Geometry: final body of the model. Coordinates: model frame, mm. Face numbers are marked on the shaded views. A direction names the side the tool comes from. Coordinates: 2 decimals unless noted, no trailing zeros. Order: outer loops, then holes, each group sorted by start corner. A loop starts at its lowest first (then second) coordinate and runs counter-clockwise, first axis right, second up. Notation, with made-up numbers: (-6, 59.5) -> (34, 59.5) arc R16 cw to (34, 85.5) -> close; hole circle Ø2 at (14, 36.25). An arc over 180 degrees is marked (long way). Answer in a Markdown table with one row per item. Add a question column.
1) Contact query for flat-ended pins moving along their axis: P1, Ø1.5, axis at x = 1.5, y = 41.5, coming from the -Z side; P2, Ø15, axis at y = 50, z = 21.5, coming from the -X side; P3, Ø9, axis at y = 52, z = 28, coming from the +X side; P4, Ø4.5, axis at x = 39.94, z = -5.63, coming from the -Y side. Output: stop coordinate, or through.
2) Pull-direction query (Z, two-part tool) for the marked faces 1, 2 and 3; classes: +Z half, -Z half, draft (parallel to the pull), parting line (faces both ways), or undercut.
3) Section query C-C on x = 22.5. Return the cut outline in (y, z).
4) Set-up query: the marked faces 4, 5 and 6. Return all of +Z, -Z, +X, -X, +Y, -Y with unobstructed straight access to the full face (end or side cutting, diameter ignored); none if empty.
5) Ray query, line 1 (X direction, y = 16, z = 21.5); line 2 (X direction, y = 8, z = -7); line 3 (Z direction, x = -11, y = 34.5). Return the intervals inside material, ascending. Write a range as from..to.
6) Section query A-A on z = 7.5. Return the cut outline in (x, y), then the cut area to 3 significant figures.
7) Section query B-B on y = 23. Return the cut outline in (x, z), then the cut area to 3 significant figures.
8) Section query D-D on y = 9. Return the cut outline in (x, z).
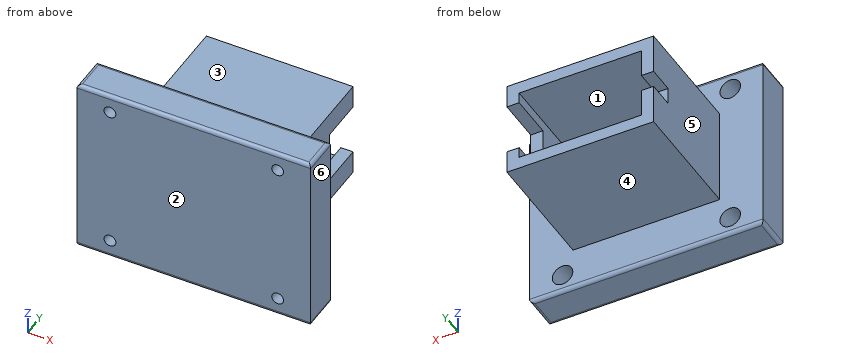
```python
from build123d import *

# Parameters (mm, degrees)
SKETCH_1_W          = 95.6
SKETCH_1_H          = 75
SKETCH_1_R          = 2.415
EXTRUDE_1_DEPTH     = 15
FILLET_1_R          = 1.5
SKETCH_2_W          = 60
SKETCH_2_H          = 40
SKETCH_2_W_2        = 50
SKETCH_2_H_2        = 30
EXTRUDE_2_DEPTH     = 50
SKETCH_3_R          = 4.2
CUT_EXTRUDE_1_DEPTH = 10.5
SKETCH_5_W          = 21
SKETCH_5_H          = 18
CUT_EXTRUDE_2_DEPTH = 5
SKETCH_6_W          = 7
SKETCH_6_H          = 11
CUT_EXTRUDE_3_DEPTH = 5


with BuildPart() as part:
    # 草圖1 → 填料-伸長1 (new body)
    with BuildSketch(Plane(origin=(0, 0, 0), x_dir=(1, 0, 0), z_dir=(0, 1, 0))):
        with Locations((5.640991766, -24.322966942)):
            Rectangle(SKETCH_1_W, SKETCH_1_H)
        with Locations(Location((-28.659008234, -54.272966942, 0), (0, 0, 270))):
            Circle(SKETCH_1_R, mode=Mode.SUBTRACT)
        with Locations(Location((-28.659008234, 5.627033058, 0), (0, 0, 270))):
            Circle(SKETCH_1_R, mode=Mode.SUBTRACT)
        with Locations(Location((39.940991766, 5.627033058, 0), (0, 0, 270))):
            Circle(SKETCH_1_R, mode=Mode.SUBTRACT)
        with Locations(Location((39.940991766, -54.272966942, 0), (0, 0, 270))):
            Circle(SKETCH_1_R, mode=Mode.SUBTRACT)
    extrude(amount=EXTRUDE_1_DEPTH)

    # 圓角1
    fillet_1_edges = [part.edges().sort_by_distance(p)[0] for p in [
        (5.640991766, 15, -13.177033058),
        (5.640991766, 0, -13.177033058),
        (5.640991766, 0, 61.822966942),
        (-42.159008234, 7.5, -13.177033058),
        (53.440991766, 7.5, -13.177033058),
        (53.440991766, 7.5, 61.822966942),
        (-42.159008234, 7.5, 61.822966942),
        (5.640991766, 15, 61.822966942),
    ]]
    fillet(fillet_1_edges, radius=FILLET_1_R)

    # 草圖2 → 填料-伸長2 (add)
    with BuildSketch(Plane(origin=(0, 15, 0), x_dir=(1, 0, 0), z_dir=(0, 1, 0))):
        with Locations((5.640991766, -24.322966942)):
            Rectangle(SKETCH_2_W, SKETCH_2_H)
        with Locations((5.640991766, -24.322966942)):
            Rectangle(SKETCH_2_W_2, SKETCH_2_H_2, mode=Mode.SUBTRACT)
    extrude(amount=EXTRUDE_2_DEPTH)

    # 草圖3 → 除料-伸長1 (cut)
    with BuildSketch(Plane(origin=(0, 15, 0), x_dir=(1, 0, 0), z_dir=(0, 1, 0))):
        with Locations(Location((-28.659008234, 5.627033058, 0), (0, 0, 270))):
            Circle(SKETCH_3_R)
        with Locations(Location((39.940991766, 5.627033058, 0), (0, 0, 270))):
            Circle(SKETCH_3_R)
        with Locations(Location((39.940991766, -54.272966942, 0), (0, 0, 270))):
            Circle(SKETCH_3_R)
        with Locations(Location((-28.659008234, -54.272966942, 0), (0, 0, 270))):
            Circle(SKETCH_3_R)
    extrude(amount=-CUT_EXTRUDE_1_DEPTH, mode=Mode.SUBTRACT)

    # 草圖5 → 除料-伸長2 (cut)
    with BuildSketch(Plane(origin=(35.640991766, 0, 0), x_dir=(0, 0, -1), z_dir=(1, 0, 0))):
        with Locations((-24.322966942, 56)):
            Rectangle(SKETCH_5_W, SKETCH_5_H)
    extrude(amount=-CUT_EXTRUDE_2_DEPTH, mode=Mode.SUBTRACT)

    # 草圖6 → 除料-伸長3 (cut)
    with BuildSketch(Plane.ZY.offset(24.359008234)):
        with Locations((24.322966942, 59.5)):
            Rectangle(SKETCH_6_W, SKETCH_6_H)
    extrude(amount=-CUT_EXTRUDE_3_DEPTH, mode=Mode.SUBTRACT)


solid = part.part
```
Result:
| question | item | result |
|---|---|---|
| 1 | P1 | z = 4.32 |
| 1 | P2 | x = -24.36 |
| 1 | P3 | x = -19.36 |
| 1 | P4 | through |
| 2 | face 1 | undercut |
| 2 | face 2 | draft |
| 2 | face 3 | +Z half |
| 3 | outline | (0, -11.68) arc R1.5 ccw to (1.5, -13.18) -> (13.5, -13.18) arc R1.5 ccw to (15, -11.68) -> (15, 4.32) -> (65, 4.32) -> (65, 9.32) -> (15, 9.32) -> (15, 39.32) -> (65, 39.32) -> (65, 44.32) -> (15, 44.32) -> (15, 60.32) arc R1.5 ccw to (13.5, 61.82) -> (1.5, 61.82) arc R1.5 ccw to (0, 60.32) -> close |
| 4 | face 4 | -Z, +X, -X, +Y |
| 4 | face 5 | +Z, -Z, -X, +Y |
| 4 | face 6 | +Z, -Z, +X, +Y, -Y |
| 5 | line 1 | -24.36..-19.36, 30.64..35.64 |
| 5 | line 2 | -42.16..-32.63, -24.69..35.97, 43.91..53.44 |
| 5 | line 3 | 4.32..9.32, 39.32..44.32 |
| 6 | outline | (-42.16, 0) -> (53.44, 0) -> (53.44, 15) -> (35.64, 15) -> (35.64, 65) -> (-24.36, 65) -> (-24.36, 15) -> (-42.16, 15) -> close |
| 6 | area | 4,430 mm2 |
| 7 | outline | (-24.36, 4.32) -> (35.64, 4.32) -> (35.64, 44.32) -> (-24.36, 44.32) -> close; hole (-19.36, 9.32) -> (30.64, 9.32) -> (30.64, 39.32) -> (-19.36, 39.32) -> close |
| 7 | area | 900 mm2 |
| 8 | outline | (-42.16, -11.68) arc R1.5 ccw to (-40.66, -13.18) -> (51.94, -13.18) arc R1.5 ccw to (53.44, -11.68) -> (53.44, 60.32) arc R1.5 ccw to (51.94, 61.82) -> (-40.66, 61.82) arc R1.5 ccw to (-42.16, 60.32) -> close; hole circle Ø8.4 at (-28.66, -5.63); hole circle Ø8.4 at (-28.66, 54.27); hole circle Ø8.4 at (39.94, -5.63); hole circle Ø8.4 at (39.94, 54.27) |
